The model under review builds one solid part; all positions refer to its coordinate system, in mm. Round coordinates to 2 decimals unless told otherwise and drop trailing zeros. Order: outer loops, then holes, each group sorted by start corner. A loop starts at its lowest first (then second) coordinate and runs counter-clockwise, first axis right, second up. Notation, with made-up numbers: M -37.5,73.5 L -1.5,73.5 A38 cw -1.5,112.5 Z; hole C 51,59 d5. An arc over 180 degrees is marked long. Answer as a JSON object with one key per item and string values. Group by question number.
1. Clearance check with flat-ended pins moving along their axes: P1, Ø6, axis at y = -15.5, z = 5.5, coming from the +X side; P2, Ø2, axis at x = -25, z = 3, coming from the +Y side; P3, Ø5, axis at y = -38.5, z = 1, coming from the -X side. State where each tip first meets the part, or that it passes through.
2. Add section C-C on z = 7.25. State the section outline as (x, y) points, and give its area (3 significant figures).
3. Mouldability with a two-part tool opening along Y and no side actions: class faces 1 (the face through (-14.985, 0.66, 8.028)), 2 (the face through (10, 12, 10)), 3 (the face through (47.69, 15.02, 4.94)), 4 (the face through (0, 0, 6)) as released by +Y, released by -Y, zero draft, split by the parting line, or undercut.
4. To check wall thickness, follow probe 1 along Y at (x, z) = (0, 9); probe 2 along Z at (x, y) = (-3, 5); probe 3 along Y at (x, z) = (-42, 7.5). State the ranges of each line that lie inside material, in increasing order. Write a range as [from, to].
5. Add section A-A on x = 0. State the section outline as (y, z) points.
```python
from build123d import *

# Parameters (mm, degrees)
F0_R     = 50
F1_DEPTH = 10
F2_R     = 15
F3_DEPTH = 4
F4_SIZE  = 1


with BuildPart() as f1:
    # F0 (on Top) → F1 (new body)
    with BuildSketch(Plane.XY):
        Circle(F0_R)
    extrude(amount=F1_DEPTH)

    # F2 (on face) → F3 (cut)
    with BuildSketch(Plane.XY.offset(10)):
        Circle(F2_R)
    extrude(amount=-F3_DEPTH, mode=Mode.SUBTRACT)

    # F4
    f4_edges = [f1.edges().sort_by_distance(p)[0] for p in [
        (-50, 0, 10),
        (-50, 0, 0),
    ]]
    chamfer(f4_edges, length=F4_SIZE)


solid = f1.part
```
Recorded:
{
 "1": {"P1": "stops at x = 48.41", "P2": "stops at y = 43.86", "P3": "stops at x = -34.7"},
 "2": {"outline": "C 0,0 d100; hole C 0,0 d30", "area": "7,150 mm²"},
 "3": {"face 1": "undercut", "face 2": "zero draft", "face 3": "split by the parting line", "face 4": "undercut"},
 "4": {"probe 1": "y = [-50, -15], [15, 50]", "probe 2": "z = [0, 6]", "probe 3": "y = [-27.13, 27.13]"},
 "5": {"outline": "M -50,1 L -49,0 L 49,0 L 50,1 L 50,9 L 49,10 L 15,10 L 15,6 L -15,6 L -15,10 L -49,10 L -50,9 Z"}
}
